Check sheet for the modelled part. Datum: model origin and axes. Units: mm. Face numbers are marked on the shaded views. A direction names the side the tool comes from. Round coordinates to 2 decimals unless told otherwise and drop trailing zeros. Order: outer loops, then holes, each group sorted by start corner. A loop starts at its lowest first (then second) coordinate and runs counter-clockwise, first axis right, second up. Notation, with made-up numbers: (36, 89.25) -> (52, 89.25) arc R22 ccw to (52, 128.25) -> close; hole circle Ø6 at (86, -8.75). An arc over 180 degrees is marked (long way). Answer in a Markdown table with one row per item. Add a question column.
1. Sectioned sample at D-D, the plane x = 101. Record the boundary of the cut face in (y, z) (3 decimals), then the cut area to 3 significant figures.
2. Access from +Z, -Z, +X, -X, +Y, -Y to the whole of each face (thin tool, end or side, straight path). Record for the marked faces 1, 2, 3 and 4.
3. Sectioned sample at B-B, the plane y = 24. Record the boundary of the cut face in (x, z) (3 decimals).
4. Sectioned sample at A-A, the plane x = 14. Record the boundary of the cut face in (y, z) (1 decimal), then the cut area to 3 significant figures.
5. Depth check by flat-ended pin: P1, Ø10, axis at y = 27.5, z = 11.5, coming from the +X side; P2, Ø6, axis at x = 113, z = 8.5, coming from the +Y side; P3, Ø2, axis at y = 61.5, z = 18.5, coming from the +X side. Enter the tip coordinate at first touch or a pass-through.
6. Material ranges on L1, parallel to Z at x = 149, y = 89 (3 decimals); L2, parallel to X at y = 63, z = 23.5, recorded low to high. Write a range as from..to.
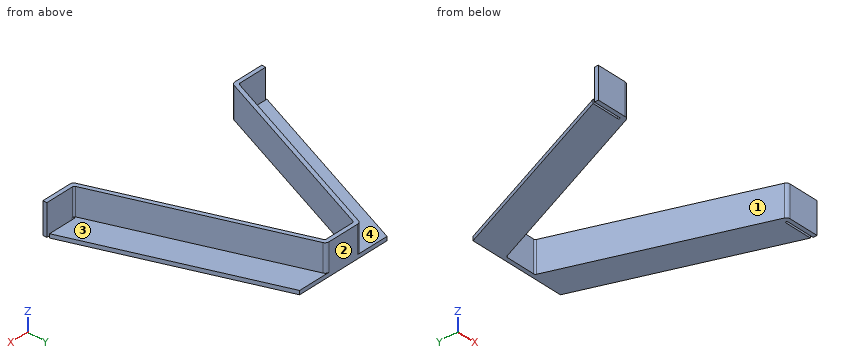
Autodesk Inventor part; units mm, degrees
ref_plane "YZ Plane" through (0, 0, 0) normal (1, 0, 0) x (0, 1, 0)
ref_plane "XZ Plane" through (0, 0, 0) normal (0, 1, 0) x (-1, 0, 0)
ref_plane "XY Plane" through (0, 0, 0) normal (0, 0, 1) x (1, 0, 0)
sketch "Sketch1" plane through (0, 0, 0) normal (0, 0, 1) x (1, 0, 0)
  line L0 (0, 0) -> (193.675, 0)
  line L1 (84.1375, 152.4) -> (109.5375, 152.4)
  line L2 (84.1375, 152.4) -> (25.9752, 0)
  line L3 (109.5375, 152.4) -> (167.6998, 0)
  line L4 (58.1623, 155.575) -> (0.6059, 4.7625)
  line L5 (135.5127, 155.575) -> (193.0691, 4.7625)
  line L6 (0, 0) -> (0, 3.175)
  line L7 (0, 3.175) -> (23.7885, 3.175)
  line L8 (193.675, 0) -> (193.675, 3.175)
  line L9 (193.675, 3.175) -> (169.8865, 3.175)
  line L10 (169.8865, 3.175) -> (111.7241, 155.575)
  line L11 (111.7241, 155.575) -> (81.9509, 155.575)
  line L12 (81.9509, 155.575) -> (23.7885, 3.175)
  line L13 (58.1623, 155.575) -> (81.9509, 155.575)
  line L14 (111.7241, 155.575) -> (135.5127, 155.575)
  line L15 (0.6059, 4.7625) -> (22.3923, 4.7625)
  line L16 (193.0691, 4.7625) -> (171.2827, 4.7625)
  arc A0 (22.3923, 3.175) -> (22.3923, 4.7625) centre (22.3923, 3.9688) ccw
  arc A1 (171.2827, 4.7625) -> (171.2827, 3.175) centre (171.2827, 3.9688) ccw
  dimension "d0" = 193.675
  dimension "d1" = 25.4
  dimension "d2" = 25.4
  dimension "d3" = 25.4
  dimension "d4" = 3.175
  dimension "d5" = 3.175
  dimension "d6" = 152.4
  dimension "d7" = 1.5875
  dimension "d8" = 1.5875
  dimension "d9" = 1.5875
extrude "Extrusion1" add sketch "Sketch1" along normal blind 25.4 contours L6 L7 L12 L11 L10 L9 L8 L0 L3 L1 L2
extrude "Extrusion2" add sketch "Sketch1" along normal blind 3.175 contours A0 L15 L4 L13 L12 L7 | L9 L10 L14 L5 L16 A1
fillet "Fillet1" radius 1.5875 4 edges at (169.8865, 3.175, 14.2875) (23.7885, 3.175, 14.2875) (84.1375, 152.4, 12.7) (109.5375, 152.4, 12.7)
fillet "Fillet2" radius 3.175 4 edges at (81.9509, 155.575, 14.2875) (111.7241, 155.575, 14.2875) (25.9752, 0, 12.7) (167.6998, 0, 12.7)
equation "\"d5\" = d4"
equation "\"d7\" = 0.5 * d4"
equation "\"d9\" = d8"
properties part number "bunny throw base 2"
Answer key:
| question | item | result |
|---|---|---|
| 1 | outline | (152.4, 0) -> (155.575, 0) -> (155.575, 25.4) -> (152.4, 25.4) -> close |
| 1 | area | 80.6 mm² |
| 2 | face 1 | +Z, -Z, -Y |
| 2 | face 2 | +Z, -Z, +X, -X, +Y |
| 2 | face 3 | +Z, +X, +Y |
| 2 | face 4 | +Z, -X, +Y |
| 3 | outline | (7.948, 0) -> (35.135, 0) -> (35.135, 25.4) -> (31.736, 25.4) -> (31.736, 3.175) -> (7.948, 3.175) -> close; (158.54, 0) -> (185.727, 0) -> (185.727, 3.175) -> (161.939, 3.175) -> (161.939, 25.4) -> (158.54, 25.4) -> close |
| 4 | outline | (0, 0) -> (3.2, 0) -> (3.2, 25.4) -> (0, 25.4) -> close; (4.8, 0) -> (39.9, 0) -> (39.9, 3.2) -> (4.8, 3.2) -> close |
| 4 | area | 192 mm² |
| 5 | P1 | stops at x = 162.51 |
| 5 | P2 | stops at y = 155.54 |
| 5 | P3 | stops at x = 148.01 |
| 6 | L1 | z = 0..3.175 |
| 6 | L2 | x = 46.62..50.02, 143.66..147.05 |
